Design review of the part built by this model. Coordinates are the model's own, in mm. Face numbers are marked on the shaded views. A direction names the side the tool comes from. Coordinates: 2 decimals unless noted, no trailing zeros. Write each loop counter-clockwise with the first axis right and the second up, starting at its lowest first coordinate (ties: lowest second). Pieces come first, ordered by that corner, then holes. Notation, with made-up numbers: (11, 77.25) -> (30, 77.25) arc R14 cw to (30, 92.25) -> close; hole circle Ø10 at (-37.75, 60). An arc over 180 degrees is marked (long way). Answer in a Markdown table with one row per item. Add a question column.
Item 1: To check wall thickness, follow line 1 (Z direction, x = 209, y = 317); line 2 (X direction, y = -211.5, z = 378); line 3 (Z direction, x = 510.5, y = -340). State the ranges of each line that lie inside material, in increasing order.
Item 2: Take a section at D-D, the plane y = 110. Write out the cut boundary in (x, z), and give its area (3 significant figures).
Item 3: Take a section at A-A, the plane x = 32.5. Write out the cut boundary in (y, z), and give its area (3 significant figures).
Item 4: Draft analysis for pull direction Z (two halves, no side actions). For the marked faces 1, 2 and 3, state which applies: released by +Z, released by -Z, zero draft, split by the parting line, or undercut.
Item 5: Clearance check with flat-ended pins moving along their axes: P1, Ø12, axis at x = -536.5, z = 601, coming from the -Y side; P2, Ø6, axis at x = 328, y = -100, coming from the -Z side; P3, Ø8, axis at x = 245.5, z = 503, coming from the +Y side. State where each tip first meets the part, or that it passes through.
Item 6: Take a section at B-B, the plane y = -189. Write out the cut boundary in (x, z).
Item 7: For the marked faces 4, 5 and 6, list the 3-axis set-ups (+Z, -Z, +X, -X, +Y, -Y) from which the entire face can be reached by the end or side of a thin tool; tool diameter is ignored.
Item 8: Take a section at C-C, the plane z = 659. Write out the cut boundary in (x, y), and give its area (3 significant figures).
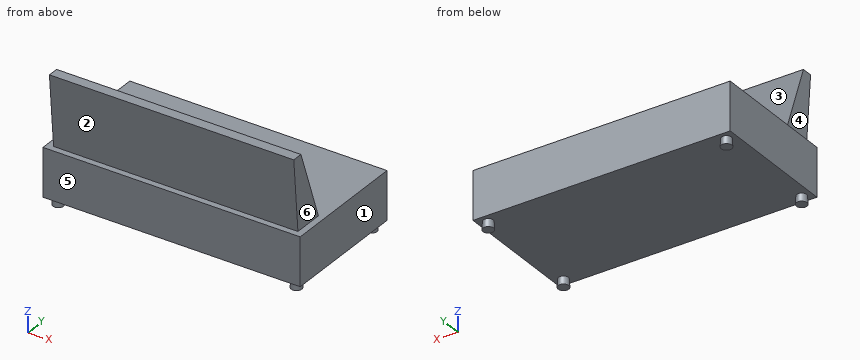
from build123d import *

# Parameters (mm, degrees)
F0_W     = 1600
F0_H     = 800
F1_DEPTH = 300
F2_R     = 30.5098573856
F3_DEPTH = 50
F3_TAPER = -3
F5_DEPTH = 760


with BuildPart() as f1:
    # F0 (on Top) → F1 (new body)
    with BuildSketch(Plane.XY):
        Rectangle(F0_W, F0_H)
    extrude(amount=F1_DEPTH)

    # F2 (on face) → F3 (join)
    with BuildSketch(Plane(origin=(0, 0, 0), x_dir=(1, 0, 0), z_dir=(0, 0, -1))):
        with Locations((-740.8549189568, -346.6182351112)):
            Circle(F2_R)
        with Locations((740.8549189568, -346.6182351112)):
            Circle(F2_R)
        with Locations((740.8549189568, 346.6182351112)):
            Circle(F2_R)
        with Locations((-740.8549189568, 346.6182351112)):
            Circle(F2_R)
    extrude(amount=F3_DEPTH, taper=F3_TAPER)

    # F4 (on Right) → F5 (join, symmetric)
    with BuildSketch(Plane.YZ):
        Polygon((-355.8277244632, 230.5950983165), (-157.0006990349, 254.912089853), (-334.2544257721, 750), (-400, 750), align=None)
    extrude(amount=F5_DEPTH, both=True)


solid = f1.part
Answers:
| question | item | result |
|---|---|---|
| 1 | line 1 | z = 0 to 300 |
| 1 | line 2 | x = -760 to 760 |
| 1 | line 3 | z = 0 to 750 |
| 2 | outline | (-800, 0) -> (800, 0) -> (800, 300) -> (-800, 300) -> close |
| 2 | area | 480,000 mm^2 |
| 3 | outline | (-400, 0) -> (400, 0) -> (400, 300) -> (-173.14, 300) -> (-334.25, 750) -> (-400, 750) -> (-361.73, 300) -> (-400, 300) -> close |
| 3 | area | 297,000 mm^2 |
| 4 | face 1 | zero draft |
| 4 | face 2 | undercut |
| 4 | face 3 | released by +Z |
| 5 | P1 | stops at y = -387.84 |
| 5 | P2 | stops at z = 0 |
| 5 | P3 | stops at y = -244.39 |
| 6 | outline | (-800, 0) -> (800, 0) -> (800, 300) -> (760, 300) -> (760, 344.29) -> (-760, 344.29) -> (-760, 300) -> (-800, 300) -> close |
| 7 | face 4 | +Z, -X, +Y, -Y |
| 7 | face 5 | +Z, -Z, +X, -X, -Y |
| 7 | face 6 | +Z, +X, +Y, -Y |
| 8 | outline | (-760, -392.26) -> (760, -392.26) -> (760, -301.67) -> (-760, -301.67) -> close |
| 8 | area | 138,000 mm^2 |
